Verification items for the finished model (mm, model axes). A direction names the side the tool comes from. Give positions to 0.01 mm unless a question says otherwise; leave off trailing zeros. Write item = value, one per line.
from build123d import *

# Parameters (mm, degrees)
F1_DEPTH = 7
F2_COUNT = 5
F3_SIZE  = 3.49999


# Not quite as in the source:
# - a fillet or chamfer is up to 0.001 mm smaller than in the source, because OpenCascade refuses the exact size


with BuildPart() as f1:
    # F0 (on Top) → F1 (new body)
    with BuildSketch(Plane.XY):
        Polygon((-12.124355653, 11.8902331595), (12.124355653, 11.8902331595), (0, 32.8902331595), align=None)
        with BuildLine():
            Line((7, 3.0145888124), (12.124355653, 11.8902331595))
            Line((12.124355653, 11.8902331595), (-12.124355653, 11.8902331595))
            Line((-12.124355653, 11.8902331595), (-7, 3.0145888124))
            ThreePointArc((-7, 3.0145888124), (0, 4.8902331595), (7, 3.0145888124))
        make_face()
        with BuildLine():
            Line((5.5125, 0.4381632362), (7, 3.0145888124))
            ThreePointArc((7, 3.0145888124), (0, 4.8902331595), (-7, 3.0145888124))
            Line((-7, 3.0145888124), (-5.5125, 0.4381632362))
            ThreePointArc((-5.5125, 0.4381632362), (0, 1.9152331595), (5.5125, 0.4381632362))
        make_face()
        with BuildLine():
            ThreePointArc((14, -9.1097668405), (12.124355653, -2.1097668405), (7, 3.0145888124))
            Line((7, 3.0145888124), (5.5125, 0.4381632362))
            ThreePointArc((5.5125, 0.4381632362), (9.5479300767, -3.5972668405), (11.025, -9.1097668405))
            ThreePointArc((11.025, -9.1097668405), (-5.5125, -18.6576969173), (-5.5125, 0.4381632362))
            Line((-5.5125, 0.4381632362), (-7, 3.0145888124))
            ThreePointArc((-7, 3.0145888124), (-7, -21.2341224935), (14, -9.1097668405))
        make_face()
    extrude(amount=F1_DEPTH)

    # F2: F1 ×5 about axis
    f2_axis = Axis((0, -9.1097668405, 0), (0, 0, -1))


with BuildPart() as f1_1:
    add(f1.part)
    for i in range(1, F2_COUNT):
        add(f1.part.rotate(f2_axis, i * 360 / F2_COUNT))

    # F3 (size 3.5 in the source; OpenCascade refuses exactly that, so slightly less here)
    f3_edges = [f1_1.edges().sort_by_distance(p)[0] for p in [
        (-13.610831, -38.157061, 7),
        (-23.41964, -31.030543, 7),
        (-18.706443, -13.085944, 7),
        (-17.470968, -16.888343, 7),
        (-31.831596, -5.141205, 7),
        (-28.084964, 6.389742, 7),
        (-9.562178, 7.452411, 7),
        (-12.796692, 5.102399, 7),
        (-6.062178, 22.390233, 7),
        (6.062178, 22.390233, 7),
        (9.562178, 7.452411, 7),
        (12.796692, 5.102399, 7),
        (28.084964, 6.389742, 7),
        (31.831596, -5.141205, 7),
        (18.706443, -13.085944, 7),
        (17.470968, -16.888343, 7),
        (23.41964, -31.030543, 7),
        (13.610831, -38.157061, 7),
        (1.99904, -28.129357, 7),
        (-1.99904, -28.129357, 7),
        (-13.610831, -38.157061, 0),
        (-23.41964, -31.030543, 0),
        (-1.99904, -28.129357, 0),
        (1.99904, -28.129357, 0),
        (13.610831, -38.157061, 0),
        (23.41964, -31.030543, 0),
        (17.470968, -16.888343, 0),
        (18.706443, -13.085944, 0),
        (31.831596, -5.141205, 0),
        (28.084964, 6.389742, 0),
        (12.796692, 5.102399, 0),
        (9.562178, 7.452411, 0),
        (6.062178, 22.390233, 0),
        (-6.062178, 22.390233, 0),
        (-9.562178, 7.452411, 0),
        (-12.796692, 5.102399, 0),
        (-28.084964, 6.389742, 0),
        (-31.831596, -5.141205, 0),
        (-18.706443, -13.085944, 0),
        (-17.470968, -16.888343, 0),
    ]]
    chamfer(f3_edges, length=F3_SIZE)


solid = f1_1.part
1) Depth check by flat-ended pin: P1, Ø1, axis at x = -12.5, z = 5.5, coming from the -Y side; P2, Ø8, axis at x = 25.5, y = -32.5, coming from the +Z side; P3, Ø2, axis at x = 13.5, z = 2.5, coming from the -Y side. Enter the tip coordinate at first touch or a pass-through.
From the geometry:
P1 = -36.06
P2 = 5.58
P3 = -38.19
2) Draft check along Y on faces 1 (the flat face through (4.65, 21.38, 1.77)), 2 (the flat face through (-14.468, -36.65, 5.226)), 3 (the flat face through (7.919, 8.058, 1.774)). Enter one of: +Y half, -Y half, draft (parallel to the pull), parting line (faces both ways), or undercut.
From the geometry:
face_1 = +Y half
face_2 = -Y half
face_3 = undercut
3) Tool access check on faces 4 (the flat face through (-7.99, 8.19, 1.77)), 5 (the flat face through (-21.686, -31.042, 1.774)), 6 (the flat face through (3.684, -27.653, 1.774)). Record the directions out of +Z, -Z, +X, -X, +Y, -Y that give a thin tool (end or side, any length) a straight path to the whole face; none if there is none.
From the geometry:
face_4 = -Z
face_5 = -Z, -X
face_6 = -Z, -Y
4) Material ranges on probe 1 along X at (y, z) = (-13.5, 1.25); probe 2 along X at (y, z) = (-30.5, 6.25); probe 3 along Y at (x, z) = (-15, 4.25), recorded low to high. Write a range as from..to.
From the geometry:
probe_1 = -13.29..-10.11, 10.11..13.29
probe_2 = -20.6..-5.01, 5.01..20.6
probe_3 = -37.95..-16.61, -11.53..6.43
